Input: part model. Units: mm. Frame: model coordinates. A direction names the side the tool comes from. Coordinates: 2 decimals unless noted, no trailing zeros. Write each loop counter-clockwise with the first axis right and the second up, starting at its lowest first coordinate (ties: lowest second). Pieces come first, ordered by that corner, then holes.
1) Pin query (flat end, axial travel): pin 1 Ø4 at (x, z) = (37, 8.5) entering from -Y. Return the tip coordinate at first contact, or that it passes through.
2) Section query B-B (x = 43). Output: boundary loops of the cut face in (y, z), then the cut area to 3 significant figures.
3) Section query A-A (z = 30). Output: boundary loops of the cut face in (x, y), then the cut area to 3 significant figures.
4) Line query: L1, parallel to X at y = -73, z = 16; L2, parallel to Z at x = 14.5, y = -69; L3, parallel to Z at x = 34, y = -71. Output: solid intervals per line, ascending.
5) Set-up query: faces 1 (the flat face through (-10, -76.2, -18)), 2 (the flat face through (6.306, -47, 27)). Return all of +Z, -Z, +X, -X, +Y, -Y with unobstructed straight access to the full face (end or side cutting, diameter ignored); none if empty.
6) Section query C-C (y = -34). Output: boundary loops of the cut face in (x, z), then the cut area to 3 significant figures.
from build123d import *

# Parameters (mm, degrees)
F0_W     = 108.6415843582
F0_H     = 101.6
F1_DEPTH = 76.2
F2_W     = 76.2
F2_H     = 43.6811229765
F3_DEPTH = 50.8
F5_DEPTH = 50.8


with BuildPart() as f1:
    # F0 (on Front) → F1 (new body)
    with BuildSketch(Plane.XZ):
        with Locations((2.785647288, -7.1188770235)):
            Rectangle(F0_W, F0_H)
    extrude(amount=F1_DEPTH)

    # F2 (on face) → F3 (cut)
    with BuildSketch(Plane.YZ.offset(57.1064394671)):
        with Locations((-38.1, 21.8405614883)):
            Rectangle(F2_W, F2_H)
    extrude(amount=-F3_DEPTH, mode=Mode.SUBTRACT)

    # F4 (on face) → F5 (join)
    with BuildSketch(Plane.YZ.offset(6.3064394671)):
        Polygon((0, 0), (0, 41.0109274089), (-76.2, 0), align=None)
    extrude(amount=F5_DEPTH)


solid = f1.part
Answer:
1. pin 1: stops at y = -64.12
2. outline: (-76.2, -57.92) - (0, -57.92) - (0, 41.01) - (-76.2, 0) - close
2. area: 5,980 mm2
3. outline: (-51.54, -76.2) - (6.31, -76.2) - (6.31, -20.46) - (57.11, -20.46) - (57.11, 0) - (-51.54, 0) - close
3. area: 5,450 mm2
4. L1: x = -51.54 to 6.31
4. L2: z = -57.92 to 3.88
4. L3: z = -57.92 to 2.8
5. face 1: +Z, -Z, +X, -X, -Y
5. face 2: +Z, +X, -Y
6. outline: (-51.54, -57.92) - (57.11, -57.92) - (57.11, 22.71) - (6.31, 22.71) - (6.31, 43.68) - (-51.54, 43.68) - close
6. area: 9,970 mm2
